Could you check a few things on this model? Use its own coordinates, in mm. A direction names the side the tool comes from. Coordinates: 2 decimals unless noted, no trailing zeros. Write each loop counter-clockwise with the first axis right and the second up, starting at its lowest first coordinate (ties: lowest second). Pieces come first, ordered by that corner, then holes.
Autodesk Inventor part; units mm, degrees
ref_plane "YZ Plane" through (0, 0, 0) normal (1, 0, 0) x (0, 1, 0)
ref_plane "XZ Plane" through (0, 0, 0) normal (0, 1, 0) x (-1, 0, 0)
ref_plane "XY Plane" through (0, 0, 0) normal (0, 0, 1) x (1, 0, 0)
sketch "Sketch1" plane through (0, 0, 0) normal (0, 0, 1) x (1, 0, 0)
  arc A0 (4, 0) -> (-4, 0) centre (0, 0) ccw
  line L0 (0, 0) -> (0, -10) construction
  line L1 (-4, 0) -> (-4, -10)
  line L2 (4, 0) -> (4, -10)
  arc A1 (-4, -10) -> (4, -10) centre (0, -10) ccw
  circle A2 centre (0, 0) radius 2
  circle A3 centre (0, -10) radius 2
  dimension "d0" = 8
  dimension "d2" = 8
  dimension "d3" = 10
  dimension "d4" = 4
  dimension "d5" = 4
extrude "Extrusion1" add sketch "Sketch1" along normal blind 2.5
sketch "Sketch4" plane through (0, 0, 0) normal (1, 0, 0) x (0, 1, 0)
  line L0 (2, 2.5) -> (2, 0)
  line L1 (-2, 2.5) -> (-2, 0)
  line L2 (2, 1.25) -> (-2, 1.25)
  line L3 (-2, 1.25) -> (-2, 2)
  line L4 (-2, 2) -> (2, 2)
  line L5 (2, 2) -> (2, 1.25)
  point P0 (0, 0)
  dimension "d14" = 1.5
revolve "Revolution1" add sketch "Sketch4" angle 360 about axis through (0, 2, 1.25) along (0, -1, 0)
sketch "Sketch5" plane through (0, 0, 0) normal (1, 0, 0) x (0, 1, 0)
  line L0 (-8, 2.5) -> (-8, 0)
  line L1 (-12, 2.5) -> (-12, 0)
  line L2 (-8, 1.25) -> (-12, 1.25)
  line L3 (-12, 1.25) -> (-12, 2)
  line L4 (-12, 2) -> (-8, 2)
  line L5 (-8, 2) -> (-8, 1.25)
  point P0 (0, 0)
  dimension "d16" = 1.5
revolve "Revolution2" add sketch "Sketch5" angle 360 about axis through (0, -8, 1.25) along (0, -1, 0)
properties part number "1-16"
1. I want a section at C-C on z = 2.3. Please give me the cut outline in (x, y), plus the area to 3 significant figures.
Verdict:
outline: (-4, -10) arc R4 ccw to (4, -10) - (4, 0) arc R4 ccw to (-4, 0) - close; hole circle Ø4 at (0, -10); hole circle Ø4 at (0, 0)
area: 105 mm2
2. I want a section at B-B on y = -10.5. Please give me the cut outline in (x, z).
Verdict:
outline: (-3.97, 0) - (-1.94, 0) - (-1.94, 2.5) - (-3.97, 2.5) - close; circle Ø1.5 at (0, 1.25); (1.94, 0) - (3.97, 0) - (3.97, 2.5) - (1.94, 2.5) - close
3. I want a section at D-D on z = 1.25. Please give me the cut outline in (x, y), plus the area to 3 significant figures.
Verdict:
outline: (-4, -10) arc R4 ccw to (4, -10) - (4, 0) arc R4 ccw to (-4, 0) - close; hole (-0.75, -11.85) - (-0.75, -8.15) arc R2 ccw to start; hole (-0.75, -1.85) - (-0.75, 1.85) arc R2 ccw to start; hole (0.75, -11.85) arc R2 ccw to (0.75, -8.15) - close; hole (0.75, -1.85) arc R2 ccw to (0.75, 1.85) - close
area: 117 mm2
4. For pin 1 (3 mm diameter, centred on x = 0, y = -10, fed in from +Z), with a flat end and sliding along its axis, tell me the tip position at first contact or that it passes through.
Verdict:
pin 1: stops at z = 2
5. I want a section at A-A on x = 1.75. Please give me the cut outline in (y, z).
Verdict:
outline: (-13.6, 0) - (-10.97, 0) - (-10.97, 2.5) - (-13.6, 2.5) - close; (-9.03, 0) - (-0.97, 0) - (-0.97, 2.5) - (-9.03, 2.5) - close; (0.97, 0) - (3.6, 0) - (3.6, 2.5) - (0.97, 2.5) - close
6. If we mould it in two halves opening along X, with no side actions, what happens to faces 3 (the face through (0, -14, 1)), 4 (the face through (1.847, 0.766, 1.232)), 5 (the face through (0, -5, 2.5))? For each: pulls with the +X half, pulls with the -X half, needs draft (parallel to the pull), parting line crosses it, or undercut.
Verdict:
face 3: parting line crosses it
face 4: undercut
face 5: needs draft
7. On a 3-axis mill with a long thin cutter (end or side, diameter ignored), from which of +Z, -Z, +X, -X, +Y, -Y can I reach the whole of each face in a straight line? I mean faces 1 (the face through (0, 4, 1)), 2 (the face through (0, 0, 0.5)). Say none if no direction works.
Verdict:
face 1: +Z, -Z, +Y
face 2: none
8. Please list where these lines run through material, in increasing order: line 1 along X through (y, z) = (-9.75, 0.8); line 2 along Y through (x, z) = (1.5, 1.65); line 3 along X through (y, z) = (-10.75, 1.3).
Verdict:
line 1: x = -4 to -1.98, -0.6 to 0.6, 1.98 to 4
line 2: y = -13.71 to -11.32, -8.68 to -1.32, 1.32 to 3.71
line 3: x = -3.93 to -1.85, -0.75 to 0.75, 1.85 to 3.93
